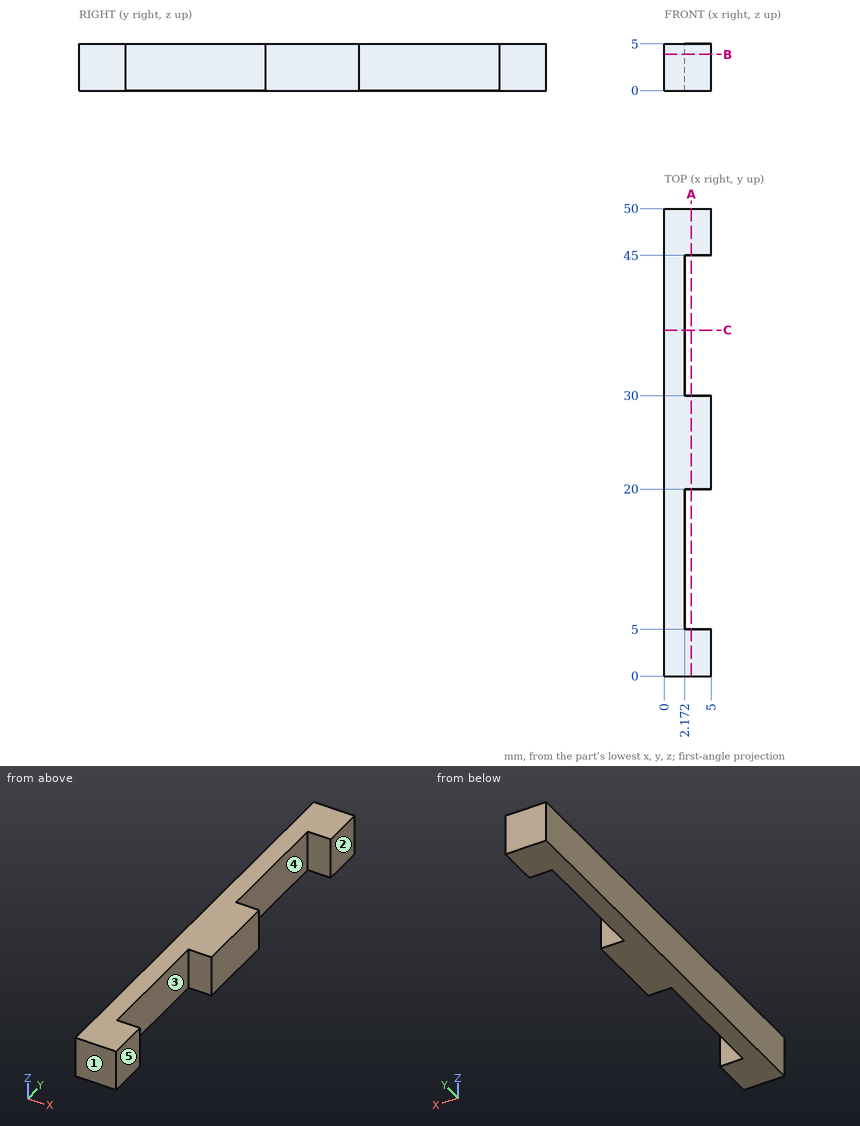
Here's the drawing with two shaded views (mm, measured from the low corner). I have some questions. A direction names the side the tool comes from. Round coordinates to 2 decimals unless told otherwise and drop trailing zeros. Loops run counter-clockwise (first coordinate to the right, second up) from the corner with the lowest first, then second, coordinate; pieces in that order, holes last. Notation, with made-up numbers: M 19.5,-26.75 L 64.5,-26.75 A20 ccw 64.5,8.25 Z; hole C -13.5,53.25 d4. An arc over 180 degrees is marked long. Answer as a JSON object with one key per item and string values. Group by question number.
Q1. Imagine slicing it at B-B, the plane z = 3.9. Please give me the cut outline in (x, y), then the cut area to 3 significant figures.
Q2. Please list where these lines run through material, in increasing order: L1, parallel to Y at x = 2.6, z = 2.8; L2, parallel to X at y = 19.5, z = 3.6.
Q3. Imagine slicing it at A-A, the plane x = 2.9. Please give me the cut outline in (y, z).
Q4. We'd pull the mould along Y, two halves only. Please class the marked faces 1, 2 and 3: +Y half, -Y half, draft (parallel to the pull), parting line (faces both ways), or undercut.
Q5. On a 3-axis mill with a long thin cutter (end or side, diameter ignored), from which of +Z, -Z, +X, -X, +Y, -Y can I reach the whole of each face in a straight line? I mean the marked faces 4 and 5. Say none if no direction works.
Q6. Will this pin go through, and if not, where does the flat tip stop? pin 1 (1.5 mm diameter, centred on y = 40.5, z = 3, fed in from +X).
Q7. Imagine slicing it at C-C, the plane y = 37. Please give me the cut outline in (x, z).
Findings:
{
 "1": {"outline": "M 0,0 L 5,0 L 5,5 L 2.17,5 L 2.17,20 L 5,20 L 5,30 L 2.17,30 L 2.17,45 L 5,45 L 5,50 L 0,50 Z", "area": "165 mm2"},
 "2": {"L1": "y = 0 to 5, 20 to 30, 45 to 50", "L2": "x = 0 to 2.17"},
 "3": {"outline": "M 0,0 L 5,0 L 5,5 L 0,5 Z; M 20,0 L 30,0 L 30,5 L 20,5 Z; M 45,0 L 50,0 L 50,5 L 45,5 Z"},
 "4": {"face 1": "-Y half", "face 2": "draft", "face 3": "undercut"},
 "5": {"face 4": "+Z, -Z, +X", "face 5": "+Z, -Z, +X, +Y, -Y"},
 "6": {"pin 1": "stops at x = 2.17"},
 "7": {"outline": "M 0,0 L 2.17,0 L 2.17,5 L 0,5 Z"}
}
